from build123d import *

# Parameters (mm, degrees)
BOSS_EXTRUDE1_DEPTH     = 30
SKETCH2_R               = 4
CUT_EXTRUDE1_DEPTH      = 41.902322672
CHAMFER1_SIZE           = 1
CUT_EXTRUDE3_DEPTH      = 41.902322672
CUT_EXTRUDE3_DEPTH_BACK = 41.902322672
SKETCH7_R               = 1.5
M4_TAPPED_HOLE1_D       = 3.3
M4_TAPPED_HOLE1_DEPTH   = 8
M4_TAPPED_HOLE1_TIP     = 0.991420021
CUT_EXTRUDE4_DEPTH      = 41.902322672


with BuildPart() as part:
    # Sketch1 → Boss-Extrude1 (new body)
    with BuildSketch(Plane.XY):
        Polygon((8, 0), (-8, 0), (-12, 4), (-16, 4), (-16, 16), (-17, 16), (-17, 22), (17, 22), (17, 16), (16, 16), (16, 4), (12, 4), align=None)
    extrude(amount=BOSS_EXTRUDE1_DEPTH)

    # Sketch2 → Cut-Extrude1 (cut, through all)
    with BuildSketch(Plane.XY.offset(30)):
        with Locations((0, 11)):
            Circle(SKETCH2_R)
    extrude(amount=-CUT_EXTRUDE1_DEPTH, mode=Mode.SUBTRACT)

    # Chamfer1
    chamfer1_edges = [part.edges().sort_by_distance(p)[0] for p in [
        (-17, 16, 15),
        (17, 16, 15),
        (-17, 22, 15),
        (17, 22, 15),
    ]]
    chamfer(chamfer1_edges, length=CHAMFER1_SIZE - 0.0001)  # a hair under: the kernel refuses the full size

    # Sketch7 → Cut-Extrude3 (cut, two sides: drawn at the far end of the back side and taken through both)
    with BuildSketch(Plane(origin=(0, 22, 0), x_dir=(1, 0, 0), z_dir=(0, 1, 0)).offset(-CUT_EXTRUDE3_DEPTH_BACK)):
        with Locations(Location((-12, -6, 0), (0, 0, 90))):
            Circle(SKETCH7_R)
        with Locations(Location((-12, -24, 0), (0, 0, 90))):
            Circle(SKETCH7_R)
        with Locations(Location((12, -6, 0), (0, 0, 90))):
            Circle(SKETCH7_R)
        with Locations(Location((12, -24, 0), (0, 0, 90))):
            Circle(SKETCH7_R)
    extrude(amount=CUT_EXTRUDE3_DEPTH + CUT_EXTRUDE3_DEPTH_BACK, mode=Mode.SUBTRACT)

    # M4 Tapped Hole1
    with Locations(Plane(origin=(0, 22, 0), x_dir=(1, 0, 0), z_dir=(0, 1, 0))):
        with Locations((-12, -6), (12, -6), (-12, -24), (12, -24)):
            Hole(M4_TAPPED_HOLE1_D / 2, depth=M4_TAPPED_HOLE1_DEPTH)
            with Locations((0, 0, -(M4_TAPPED_HOLE1_DEPTH + M4_TAPPED_HOLE1_TIP / 2))):  # 118° drill point
                Cone(0, M4_TAPPED_HOLE1_D / 2, M4_TAPPED_HOLE1_TIP, mode=Mode.SUBTRACT)

    # Sketch8 → Cut-Extrude4 (cut, through all)
    with BuildSketch(Plane(origin=(0, 0, 0), x_dir=(-1, 0, 0), z_dir=(0, 0, -1))):
        Polygon((8, 22), (3, 22), (3.2, 21.8), (7.8, 21.8), align=None)
        Polygon((-3, 22), (-8, 22), (-7.8, 21.8), (-3.2, 21.8), align=None)
    extrude(amount=-CUT_EXTRUDE4_DEPTH, mode=Mode.SUBTRACT)


solid = part.part
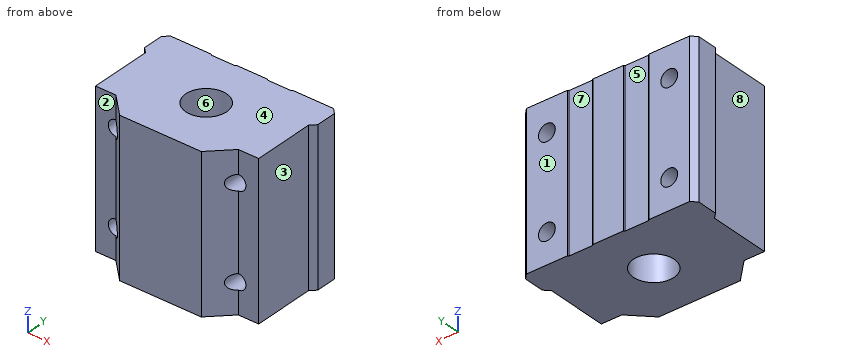
Here's how the part is built. I have some questions about the finished solid (model axes, mm). Face numbers are marked on the shaded views. A direction names the side the tool comes from. Round coordinates to 2 decimals unless told otherwise and drop trailing zeros. Order: outer loops, then holes, each group sorted by start corner. A loop starts at its lowest first (then second) coordinate and runs counter-clockwise, first axis right, second up. Notation, with made-up numbers: (80.5, 80.25) -> (84.5, 80.25) arc R20 cw to (84.5, 104.25) -> close; hole circle Ø11 at (44, 71). An arc over 180 degrees is marked (long way). Return JSON: item names as keys, results as strings.
Q1. If we mould it in two halves opening along Y, with no side actions, what happens to the marked faces 6, 7 and 8? For each: released by +Y, released by -Y, zero draft, split by the parting line, or undercut.
Filled sheet:
{"face 6": "undercut", "face 7": "released by +Y", "face 8": "zero draft"}
Q2. I need wall thicknesses on line 1 along Z through (x, y) = (12, 18.5); line 2 along Z through (x, y) = (12, 11.5); line 3 along X through (y, z) = (8.5, 24). Which ranges of each line are inside material? Lowest first, please. Write a range as from..to.
Filled sheet:
{"line 1": "z = 0..4.35, 7.65..22.35, 25.65..30", "line 2": "z = 0..4.5, 7.5..22.5, 25.5..30", "line 3": "x = -16..-13.5, -10.5..-3.12, 3.12..10.5, 13.5..16"}
Q3. If we section it at C-C on y = 20.25: List the corners of the cut face in (x, z) for me.
Filled sheet:
{"outline": "(-17, 0) -> (17, 0) -> (17, 30) -> (-17, 30) -> close; hole circle Ø3.3 at (-12, 6); hole circle Ø3.3 at (-12, 24); hole circle Ø3.3 at (12, 6); hole circle Ø3.3 at (12, 24)"}
Q4. Which directions (+Z, -Z, +X, -X, +Y, -Y) give clear straight access to the entire face, cutting with the end or side of a thin tool? Please do the marked faces 1, 2, 3, 4 and 5.
Filled sheet:
{"face 1": "+Z, -Z, +X, -X, +Y", "face 2": "+Z, -Z, -X, -Y", "face 3": "+Z, -Z, +X, -Y", "face 4": "+Z, +X, -X, +Y, -Y", "face 5": "+Z, -Z, +Y"}
Q5. For pin 1 Ø2.5 at (x, z) = (12, 24) entering from +Y; pin 2 Ø2 at (y, z) = (5, 16.5) entering from +X; pin 3 Ø3 at (x, z) = (14, 16) entering from -Y; pin 4 Ø6 at (y, z) = (12.5, 16) entering from -X, each with a flat end and sliding along its axis, tell me the tip position at first contact or that it passes through.
Filled sheet:
{"pin 1": "passes through", "pin 2": "stops at x = 16", "pin 3": "stops at y = 4", "pin 4": "stops at x = -16"}
Q6. If we section it at A-A on y = 11: List the corners of the cut face in (x, z) for me.
Filled sheet:
{"outline": "(-16, 0) -> (-4, 0) -> (-4, 30) -> (-16, 30) -> close; (4, 0) -> (16, 0) -> (16, 30) -> (4, 30) -> close; hole circle Ø3 at (-12, 6); hole circle Ø3 at (-12, 24); hole circle Ø3 at (12, 6); hole circle Ø3 at (12, 24)"}
Q7. If we section it at B-B on x = 0: List the corners of the cut face in (y, z) for me, plus the area to 3 significant figures.
Filled sheet:
{"outline": "(0, 0) -> (7, 0) -> (7, 30) -> (0, 30) -> close; (15, 0) -> (22, 0) -> (22, 30) -> (15, 30) -> close", "area": "420 mm^2"}
